Geometry check sheet. Reference: the model listing, model coordinates, mm. A direction names the side the tool comes from. Coordinates: 2 decimals unless noted, no trailing zeros. Write each loop counter-clockwise with the first axis right and the second up, starting at its lowest first coordinate (ties: lowest second). Pieces come first, ordered by that corner, then holes. Notation, with made-up numbers: (-35, 83.5) -> (-6, 83.5) arc R30 cw to (-6, 121.5) -> close; hole circle Ø4 at (-37, 4.5). An arc over 180 degrees is marked (long way). Answer in a Markdown table with one row per item. Add a question column.
Q1. Section check A-A, the plane y = 1.5. Record the boundary of the cut face in (x, z), and give its area (3 significant figures).
Q2. Gauge pin test, flat end, axial feed: P1, Ø5, axis at x = -16, y = 4, coming from the -Z side. Record the tip position at first contact, or that the pin passes through.
Q3. Section check B-B, the plane x = -12.5. Record the boundary of the cut face in (y, z) (3 decimals), and give its area (3 significant figures).
Q4. Thickness scan on line 1 (X direction, y = -6.5, z = 0.3); line 2 (X direction, y = 16.5, z = 0.4); line 3 (X direction, y = 12.5, z = 1.15). Record the ranges inside material, lowest first.
Q5. Release check for a two-part mould opening along X. For faces 3 (the face through (-10.67, 6.08, 0.79)), 4 (the face through (-20.29, -6.4, 0.79)), 5 (the face through (20.16, -6.77, 0.79)) record: pulls with the +X half, pulls with the -X half, needs draft (parallel to the pull), parting line crosses it, or undercut.
Q6. Tool access check on faces 1 (the face through (0, -21.27, 1)), 2 (the face through (-9.129, -8.213, 0.789)). Record the directions out of +Z, -Z, +X, -X, +Y, -Y that give a thin tool (end or side, any length) a straight path to the whole face; none if there is none.
Q7. Section check C-C, the plane z = 0.8. Count the separate pieces of the cut face and the enclosed holes in it, and give its area (3 significant figures).
```python
from build123d import *

# Parameters (mm, degrees)
PCB_THICKNESS_DEPTH = 1.6


with BuildPart() as part:
    # Model → PCB Thickness (new body)
    with BuildSketch(Plane.XY):
        with BuildLine():
            Line((-0.352766154, 26.023024653), (-24.647921054, 8.326484664))
            ThreePointArc((-24.647921054, 8.326484664), (-24.865455476, 8.026418687), (-24.865198885, 7.655796575))
            Line((-24.865198885, 7.655796575), (-15.584897999, -20.855706146))
            ThreePointArc((-15.584897999, -20.855706146), (-15.366905589, -21.155501644), (-15.014360333, -21.27))
            Line((-15.014360333, -21.27), (15.014062777, -21.27))
            ThreePointArc((15.014062777, -21.27), (15.366729058, -21.155413735), (15.584692966, -20.855421647))
            Line((15.584692966, -20.855421647), (24.865283806, 7.705350163))
            ThreePointArc((24.865283806, 7.705350163), (24.86528072, 8.07620295), (24.647279393, 8.376214969))
            Line((24.647279393, 8.376214969), (0.353119455, 26.023485868))
            ThreePointArc((0.353119455, 26.023485868), (0.00010165, 26.138042579), (-0.352766154, 26.023024653))
        make_face()
        with BuildLine():
            ThreePointArc((17.841223922, 8.422307775), (18.248398796, 8.899239554), (18.008187001, 9.478509434))
            Line((18.008187001, 9.478509434), (3.459163763, 20.037918253))
            ThreePointArc((3.459163763, 20.037918253), (2.833918731, 20.086966034), (2.506100046, 19.552295755))
            Line((2.506100046, 19.552295755), (2.498798945, 4.261789527))
            ThreePointArc((2.498798945, 4.261789527), (2.746033937, 3.776163066), (3.284260895, 3.69088729))
            Line((3.284260895, 3.69088729), (17.841223922, 8.422307775))
        make_face(mode=Mode.SUBTRACT)
        with BuildLine():
            ThreePointArc((-2.481000035, 19.538772626), (-2.807853844, 20.073751171), (-3.432918624, 20.025486513))
            Line((-3.432918624, 20.025486513), (-18.026854434, 9.45686058))
            ThreePointArc((-18.026854434, 9.45686058), (-18.267531635, 8.876938588), (-17.859258249, 8.399918804))
            Line((-17.859258249, 8.399918804), (-3.284491549, 3.69496499))
            ThreePointArc((-3.284491549, 3.69496499), (-2.74743143, 3.780639667), (-2.500299876, 4.265097836))
            Line((-2.500299876, 4.265097836), (-2.481000035, 19.538772626))
        make_face(mode=Mode.SUBTRACT)
        with BuildLine():
            ThreePointArc((-19.370866555, 3.544089386), (-19.978077319, 3.395006484), (-20.122996261, 2.786788494))
            Line((-20.122996261, 2.786788494), (-14.639600254, -14.089399218))
            ThreePointArc((-14.639600254, -14.089399218), (-14.164858865, -14.496276924), (-13.585986389, -14.259981534))
            Line((-13.585986389, -14.259981534), (-4.544592973, -1.993390467))
            ThreePointArc((-4.544592973, -1.993390467), (-4.456938312, -1.451989932), (-4.846077132, -1.065507257))
            Line((-4.846077132, -1.065507257), (-19.370866555, 3.544089386))
        make_face(mode=Mode.SUBTRACT)
        with BuildLine():
            ThreePointArc((13.542585003, -14.232579653), (14.121457712, -14.46887711), (14.596200254, -14.061999218))
            Line((14.596200254, -14.061999218), (20.079596261, 2.814188494))
            ThreePointArc((20.079596261, 2.814188494), (19.934677319, 3.422406484), (19.327466555, 3.571489386))
            Line((19.327466555, 3.571489386), (4.80273686, -1.038088302))
            ThreePointArc((4.80273686, -1.038088302), (4.413598402, -1.424569865), (4.50125132, -1.965969627))
            Line((4.50125132, -1.965969627), (13.542585003, -14.232579653))
        make_face(mode=Mode.SUBTRACT)
        with BuildLine():
            ThreePointArc((-9.36017471, -17.320664685), (-9.406025436, -17.9442251), (-8.872358317, -18.27))
            Line((-8.872358317, -18.27), (8.872358317, -18.27))
            ThreePointArc((8.872358317, -18.27), (9.406025435, -17.9442251), (9.36017471, -17.320664685))
            Line((9.36017471, -17.320664685), (0.487816395, -4.931187808))
            ThreePointArc((0.487816395, -4.931187808), (0, -4.680523127), (-0.487816395, -4.931187808))
            Line((-0.487816395, -4.931187808), (-9.36017471, -17.320664685))
        make_face(mode=Mode.SUBTRACT)
    extrude(amount=PCB_THICKNESS_DEPTH)


solid = part.part
```
Calculated:
| question | item | result |
|---|---|---|
| 1 | outline | (-22.86, 0) -> (-19.7, 0) -> (-19.7, 1.6) -> (-22.86, 1.6) -> close; (-12.93, 0) -> (12.8, 0) -> (12.8, 1.6) -> (-12.93, 1.6) -> close; (19.65, 0) -> (22.85, 0) -> (22.85, 1.6) -> (19.65, 1.6) -> close |
| 1 | area | 51.3 mm² |
| 2 | P1 | stops at z = 0 |
| 3 | outline | (-21.27, 0) -> (-12.787, 0) -> (-12.787, 1.6) -> (-21.27, 1.6) -> close; (1.364, 0) -> (6.67, 0) -> (6.67, 1.6) -> (1.364, 1.6) -> close; (13.459, 0) -> (17.175, 0) -> (17.175, 1.6) -> (13.459, 1.6) -> close |
| 3 | area | 28.0 mm² |
| 4 | line 1 | x = -20.26 to -17.11, -7.87 to -1.61, 1.61 to 7.84, 17.05 to 20.25 |
| 4 | line 2 | x = -13.43 to -8.3, -2.48 to 2.5, 8.33 to 13.46 |
| 4 | line 3 | x = -18.92 to -13.82, -2.49 to 2.5, 13.85 to 18.97 |
| 5 | face 3 | undercut |
| 5 | face 4 | pulls with the -X half |
| 5 | face 5 | pulls with the +X half |
| 6 | face 1 | +Z, -Z, +X, -X, -Y |
| 6 | face 2 | +Z, -Z |
| 7 | separate pieces | 1 |
| 7 | enclosed holes | 5 |
| 7 | area | 939 mm² |
